The model under review builds one solid part; all positions refer to its coordinate system, in mm. Face numbers are marked on the shaded views. A direction names the side the tool comes from. Give positions to 0.01 mm unless a question says otherwise; leave off trailing zeros. Order: outer loops, then holes, each group sorted by start corner. A loop starts at its lowest first (then second) coordinate and runs counter-clockwise, first axis right, second up. Notation, with made-up numbers: (-25.75, 20) - (32.25, 20) arc R24 ccw to (32.25, 41) - close; hole circle Ø10 at (2.5, 84). An arc over 180 degrees is marked (long way). Put each result on its own line as item: value.
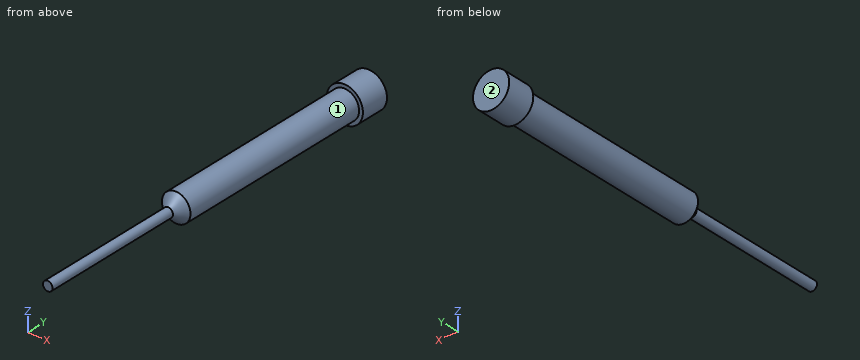
```python
from build123d import *

# Parameters (mm, degrees)
SKETCH3_R           = 0.5
BOSS_EXTRUDE4_DEPTH = 25
SKETCH5_R           = 1.5
BOSS_EXTRUDE5_DEPTH = 15
CHAMFER2_SIZE       = 10
SKETCH6_R           = 1.900672983
BOSS_EXTRUDE6_DEPTH = 3


with BuildPart() as part:
    # Sketch3 → Boss-Extrude4 (new body)
    with BuildSketch(Plane(origin=(0, 0, 0), x_dir=(1, 0, 0), z_dir=(0, 1, 0))):
        with Locations(Location((0, 0, 0), (0, 0, 270))):
            Circle(SKETCH3_R)
    extrude(amount=BOSS_EXTRUDE4_DEPTH)

    # Sketch5 → Boss-Extrude5 (add)
    with BuildSketch(Plane(origin=(0, 25, 0), x_dir=(1, 0, 0), z_dir=(0, 1, 0))):
        with Locations(Location((0, 0, 0), (0, 0, 270))):
            Circle(SKETCH5_R)
    extrude(amount=BOSS_EXTRUDE5_DEPTH)

    # Chamfer2
    # the kernel refuses this chamfer: 10 mm, written as the material it adds along each edge
    with BuildSketch(Plane(origin=(0, 25, 0), x_dir=(0, 0, 1), z_dir=(-1, 0, 0))) as chamfer2_piece_1_section:
        Polygon((0.5 + CHAMFER2_SIZE, 0), (0.5, -CHAMFER2_SIZE), (0.5, 0), align=None)
    chamfer2_piece_1 = revolve(axis=Axis((0, 25, 0), (0, 1, 0)), mode=Mode.PRIVATE)
    chamfer2_piece_1 = chamfer2_piece_1 & Plane(origin=(0, 15.387158422, 0), x_dir=(0, 0, 1), z_dir=(0, -1, 0)) * Cylinder(1.5, 42, mode=Mode.PRIVATE)
    add(chamfer2_piece_1)

    # Sketch6 → Boss-Extrude6 (add)
    with BuildSketch(Plane(origin=(0, 40, 0), x_dir=(1, 0, 0), z_dir=(0, 1, 0))):
        with Locations(Location((0, 0, 0), (0, 0, 270))):
            Circle(SKETCH6_R)
    extrude(amount=-BOSS_EXTRUDE6_DEPTH)


solid = part.part
```
(1) Take a section at B-B, the plane x = 0. Write out the cut boundary in (y, z).
The answers:
outline: (0, -0.5) - (15, -0.5) - (16, -1.5) - (37, -1.5) - (37, -1.9) - (40, -1.9) - (40, 1.9) - (37, 1.9) - (37, 1.5) - (16, 1.5) - (15, 0.5) - (0, 0.5) - close
(2) Take a section at D-D, the plane y = 22. Write out the cut boundary in (x, z), then the cut area to 3 significant figures.
The answers:
outline: circle Ø3 at (0, 0)
area: 7.07 mm^2
(3) Wall thickness on L1, parallel to Z at x = 0.1, y = 29; L2, parallel to Y at x = -1.35, z = 1.2; L3, parallel to Y at x = -0.6, z = -0.5: over which ranges is each line inside the solid? List them lowest first.
The answers:
L1: -1.5 to 1.5
L2: 37 to 40
L3: 15.28 to 40
(4) Take a section at A-A, the plane z = 0. Write out the cut boundary in (x, y), then the cut area to 3 significant figures.
The answers:
outline: (-1.9, 37) - (-1.5, 37) - (-1.5, 16) - (-0.5, 15) - (-0.5, 0) - (0.5, 0) - (0.5, 15) - (1.5, 16) - (1.5, 37) - (1.9, 37) - (1.9, 40) - (-1.9, 40) - close
area: 91.4 mm^2
(5) Take a section at C-C, the plane y = 3.5. Write out the cut boundary in (x, z).
The answers:
outline: circle Ø1 at (0, 0)
(6) Clearance check with flat-ended pins moving along their axes: pin 1 Ø1 at (x, z) = (0.5, 1) entering from -Y; pin 2 Ø2 at (y, z) = (18, -1) entering from -X; pin 3 Ø1.5 at (x, y) = (1.5, 21.5) entering from +Z. State where each tip first meets the part, or that it passes through.
The answers:
pin 1: y = 15.12
pin 2: x = -1.5
pin 3: z = 1.3
(7) For the marked faces 1 and 2, list the 3-axis set-ups (+Z, -Z, +X, -X, +Y, -Y) from which the entire face can be reached by the end or side of a thin tool; tool diameter is ignored.
The answers:
face 1: -Y
face 2: +Z, -Z, +X, -X, +Y
